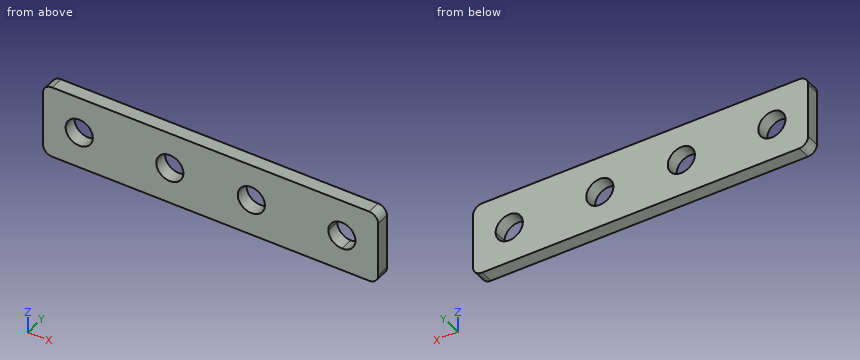
```python
from build123d import *

# Parameters (mm, degrees)
BOSS_EXTRUDE1_DEPTH = 1.5
FILLET1_R           = 1


with BuildPart() as part:
    # Sketch1 → Boss-Extrude1 (new body)
    with BuildSketch(Plane(origin=(0, 0, 0), x_dir=(1, 0, 0), z_dir=(0, 1, 0))):
        with BuildLine():
            Line((18.5, 0), (18.5, 4))
            Line((18.5, 4), (15.5, 4))
            ThreePointArc((15.5, 4), (14, 2.5), (12.5, 4))
            Line((12.5, 4), (5.5, 4))
            ThreePointArc((5.5, 4), (4, 2.5), (2.5, 4))
            Line((2.5, 4), (0, 4))
            Line((0, 4), (0, 0))
            Line((0, 0), (18.5, 0))
        make_face()
        with BuildLine():
            Line((21.5, 4), (18.5, 4))
            Line((18.5, 4), (18.5, 0))
            Line((18.5, 0), (37, 0))
            Line((37, 0), (37, 4))
            Line((37, 4), (34.5, 4))
            ThreePointArc((34.5, 4), (33, 2.5), (31.5, 4))
            Line((31.5, 4), (24.5, 4))
            ThreePointArc((24.5, 4), (23, 2.5), (21.5, 4))
        make_face()
        with BuildLine():
            Line((18.5, 4), (18.5, 8))
            Line((18.5, 8), (0, 8))
            Line((0, 8), (0, 4))
            Line((0, 4), (2.5, 4))
            ThreePointArc((2.5, 4), (4, 5.5), (5.5, 4))
            Line((5.5, 4), (12.5, 4))
            ThreePointArc((12.5, 4), (14, 5.5), (15.5, 4))
            Line((15.5, 4), (18.5, 4))
        make_face()
        with BuildLine():
            Line((33, 8), (18.5, 8))
            Line((18.5, 8), (18.5, 4))
            Line((18.5, 4), (21.5, 4))
            ThreePointArc((21.5, 4), (23, 5.5), (24.5, 4))
            Line((24.5, 4), (31.5, 4))
            ThreePointArc((31.5, 4), (31.939339828, 5.060660172), (33, 5.5))
            Line((33, 5.5), (33, 8))
        make_face()
        with BuildLine():
            Line((37, 8), (33, 8))
            Line((33, 8), (33, 5.5))
            ThreePointArc((33, 5.5), (34.060660172, 5.060660172), (34.5, 4))
            Line((34.5, 4), (37, 4))
            Line((37, 4), (37, 8))
        make_face()
    extrude(amount=BOSS_EXTRUDE1_DEPTH)

    # Fillet1
    fillet1_edges = [part.edges().sort_by_distance(p)[0] for p in [
        (0, 0.75, 0),
        (0, 0.75, -8),
        (37, 0.75, -8),
        (37, 0.75, 0),
    ]]
    fillet(fillet1_edges, radius=FILLET1_R)


solid = part.part
```
Source: CAD feature listing. Evaluate the final solid. Frame: model axes, mm. Give positions to 0.01 mm unless a question says otherwise; leave off trailing zeros. Loops run counter-clockwise (first coordinate to the right, second up) from the corner with the lowest first, then second, coordinate; pieces in that order, holes last. Notation, with made-up numbers: (-11, 85) -> (-7, 85) arc R35 cw to (-7, 121) -> close; hole circle Ø11 at (84.25, -12.5). An arc over 180 degrees is marked (long way). Use a Markdown table: item, result. Add a question column.
(1) Section query A-A (x = 14). Output: boundary loops of the cut face in (y, z).
(2) Ray query, line 1 (X direction, y = 0.6, z = -4); line 2 (X direction, y = 0.85, z = -2.75); line 3 (Z direction, x = 14, y = 0.6). Return the intervals inside material, ascending.
(3) Section query B-B (y = 0.5). Output: boundary loops of the cut face in (x, z), then the cut area to 3 significant figures.
(4) Section query D-D (z = -3). Output: boundary loops of the cut face in (x, y).
(5) First-contact query: pin 1 Ø1.8 at (x, z) = (4, -4) entering from -Y. Flat tip, straight axial feed; report the tip coordinate or a pass-through.
(6) Section query C-C (z = -4.75). Output: boundary loops of the cut face in (x, y), then the cut area to 3 significant figures.
Checked values:
| question | item | result |
|---|---|---|
| 1 | outline | (0, -8) -> (1.5, -8) -> (1.5, -5.5) -> (0, -5.5) -> close; (0, -2.5) -> (1.5, -2.5) -> (1.5, 0) -> (0, 0) -> close |
| 2 | line 1 | 0 to 2.5, 5.5 to 12.5, 15.5 to 21.5, 24.5 to 31.5, 34.5 to 37 |
| 2 | line 2 | 0 to 3.17, 4.83 to 13.17, 14.83 to 22.17, 23.83 to 32.17, 33.83 to 37 |
| 2 | line 3 | -8 to -5.5, -2.5 to 0 |
| 3 | outline | (0, -7) arc R1 ccw to (1, -8) -> (36, -8) arc R1 ccw to (37, -7) -> (37, -1) arc R1 ccw to (36, 0) -> (1, 0) arc R1 ccw to (0, -1) -> close; hole circle Ø3 at (4, -4); hole circle Ø3 at (14, -4); hole circle Ø3 at (23, -4); hole circle Ø3 at (33, -4) |
| 3 | area | 267 mm^2 |
| 4 | outline | (0, 0) -> (2.88, 0) -> (2.88, 1.5) -> (0, 1.5) -> close; (5.12, 0) -> (12.88, 0) -> (12.88, 1.5) -> (5.12, 1.5) -> close; (15.12, 0) -> (21.88, 0) -> (21.88, 1.5) -> (15.12, 1.5) -> close; (24.12, 0) -> (31.88, 0) -> (31.88, 1.5) -> (24.12, 1.5) -> close; (34.12, 0) -> (37, 0) -> (37, 1.5) -> (34.12, 1.5) -> close |
| 5 | pin 1 | through |
| 6 | outline | (0, 0) -> (2.7, 0) -> (2.7, 1.5) -> (0, 1.5) -> close; (5.3, 0) -> (12.7, 0) -> (12.7, 1.5) -> (5.3, 1.5) -> close; (15.3, 0) -> (21.7, 0) -> (21.7, 1.5) -> (15.3, 1.5) -> close; (24.3, 0) -> (31.7, 0) -> (31.7, 1.5) -> (24.3, 1.5) -> close; (34.3, 0) -> (37, 0) -> (37, 1.5) -> (34.3, 1.5) -> close |
| 6 | area | 39.9 mm^2 |
